from build123d import *

# Parameters (mm, degrees)
SKETCH2_R          = 1.160779638
CUT_EXTRUDE1_DEPTH = 7.62


with BuildPart() as part:
    # Sketch1 → Revolve1 (revolve)
    with BuildSketch(Plane(origin=(0, 0, 0), x_dir=(1, 0, 0), z_dir=(0, 1, 0))):
        Polygon((-23.567795766, 7.367626397), (-25.274044429, 9.07387506), (-26.980293092, 7.367626397), (-26.684604524, 8.778186492), (-26.684604524, 9.951033697), (-26.980293092, 9.951033697), (-26.980293092, 10.270846758), (-26.684604524, 10.270846758), (-26.684604524, 13.5627756), (-23.863484334, 13.5627756), (-23.863484334, 10.270846758), (-23.567795766, 10.270846758), (-23.567795766, 9.951033697), (-23.863484334, 9.951033697), (-23.863484334, 8.778186492), align=None)
    revolve(axis=Axis((-23.863484334, 0, -13.5627756), (1, 0, 0)))

    # Sketch2 → Cut-Extrude1 (cut)
    with BuildSketch(Plane.ZY.offset(26.684604524)):
        with Locations((-13.5627756, 0)):
            Circle(SKETCH2_R)
    extrude(amount=-CUT_EXTRUDE1_DEPTH, mode=Mode.SUBTRACT)


solid = part.part
Check sheet for the modelled part. Datum: model origin and axes. Units: mm. A direction names the side the tool comes from. Give positions to 0.01 mm unless a question says otherwise; leave off trailing zeros. Return JSON: item names as keys, results as strings. Group by question number.
1. Go/stop test with flat-tipped pins: pin 1 (5.5 mm diameter, centred on y = 1, z = -12, fed in from -X); pin 2 (3.5 mm diameter, centred on y = 0, z = -13.56, fed in from +X); pin 3 (2 mm diameter, centred on x = -26, y = -3, fed in from +Z); pin 4 (1.5 mm diameter, centred on x = -25.5, y = 1.5, fed in from -Z). Record where each tip stops, or that it passes through.
2. Tool access check on faces 1 (the flat face through (-23.863, 1.4, -13.5)), 2 (the flat face through (-26.685, -4, -13)). Record the directions out of +Z, -Z, +X, -X, +Y, -Y that give a thin tool (end or side, any length) a straight path to the whole face; none if there is none.
3. Thickness scan on L1, parallel to X at y = 2.25, z = -10.5; L2, parallel to X at y = 5, z = -13; L3, parallel to X at y = -2.5, z = -18.5. Record the ranges inside material, lowest first.
4. Mould release check, pull along X, two halves, no side actions. Record for faces 3 (the flat face through (-26.685, 1.4, -13.6)), 4 (the conical face through (-25.381, -1.38, -9.179)), 5 (the flat face through (-23.863, -4, -14)), 6 (the cylindrical face through (-25.294, 0.051, -14.722)): released by +X, released by -X, zero draft, split by the parting line, or undercut.
Return value:
{
 "1": {"pin 1": "x = -26.98", "pin 2": "x = -23.86", "pin 3": "z = -8.01", "pin 4": "z = -18.84"},
 "2": {"face 1": "+X", "face 2": "-X"},
 "3": {"L1": "-26.68 to -23.86", "L2": "-26.74 to -25.82, -24.73 to -23.81", "L3": "-26.84 to -26.32, -24.23 to -23.71"},
 "4": {"face 3": "released by -X", "face 4": "undercut", "face 5": "released by +X", "face 6": "zero draft"}
}
